Input: part model. Units: mm. Frame: model coordinates. Coordinates: 2 decimals unless noted, no trailing zeros. Write each loop counter-clockwise with the first axis right and the second up, starting at its lowest first coordinate (ties: lowest second). Pieces come first, ordered by that corner, then holes. Notation, with made-up numbers: M -11.75,19 L 14.25,19 A14 cw 14.25,37 Z; hole C -24,-26.5 d3. An arc over 180 degrees is marked long. Use one line per item in the form item = value.
from build123d import *

# Parameters (mm, degrees)
SKETCH6_W             = 25.4
SKETCH6_H             = 25.4
SKETCH6_W_2           = 20.32
SKETCH6_H_2           = 20.32
BOSS_EXTRUDE3_DEPTH   = 363.22
BOSS_EXTRUDE3_2_DEPTH = 363.22
SKETCH7_W             = 50.8
SKETCH7_H             = 25.359897542
SKETCH7_W_2           = 45.72
SKETCH7_H_2           = 20.279897542
BOSS_EXTRUDE4_DEPTH   = 114.3
CUT_EXTRUDE1_DEPTH    = 384.612481677
CUT_EXTRUDE2_DEPTH    = 384.612481677
CIRPATTERN1_COUNT     = 3
SKETCH12_R            = 3
CUT_EXTRUDE3_DEPTH    = 519.942549655
SKETCH13_R            = 87.5
BOSS_EXTRUDE6_DEPTH   = 2
SKETCH14_R            = 3
CUT_EXTRUDE4_DEPTH    = 518.180396616


with BuildPart() as part:
    # Sketch6 → Boss-Extrude3 (new body)
    with BuildSketch(Plane.XY.offset(-12.7)):
        with Locations((-44.45, 0)):
            Rectangle(SKETCH6_W, SKETCH6_H)
        with Locations((-44.45, 0)):
            Rectangle(SKETCH6_W_2, SKETCH6_H_2, mode=Mode.SUBTRACT)
    extrude(amount=-BOSS_EXTRUDE3_DEPTH)



with BuildPart() as body_2:
    # Sketch6 → Boss-Extrude3 2 (new body)
    with BuildSketch(Plane.XY.offset(-12.7)):
        with Locations((44.45, 0)):
            Rectangle(SKETCH6_W, SKETCH6_H)
        with Locations((44.45, 0)):
            Rectangle(SKETCH6_W_2, SKETCH6_H_2, mode=Mode.SUBTRACT)
    extrude(amount=-BOSS_EXTRUDE3_2_DEPTH)


with BuildPart() as part_1:
    add(part.part)

    add(body_2.part)  # Boss-Extrude4 merges body 2
    # Sketch7 → Boss-Extrude4 (add)
    with BuildSketch(Plane(origin=(-57.15, 0, 0), x_dir=(0, 0, -1), z_dir=(1, 0, 0))):
        with Locations((350.52, -25.379948771)):
            Rectangle(SKETCH7_W, SKETCH7_H)
        with Locations((350.52, -25.379948771)):
            Rectangle(SKETCH7_W_2, SKETCH7_H_2, mode=Mode.SUBTRACT)
    extrude(amount=BOSS_EXTRUDE4_DEPTH)

    # Sketch9 → Cut-Extrude1 (cut, through all)
    with BuildSketch(Plane(origin=(0, 12.7, 0), x_dir=(1, 0, 0), z_dir=(0, 1, 0))):
        Polygon((0, 0), (66.166370432, 38.20117178), (56.531711502, -13.195312554), align=None)
    extrude(amount=-CUT_EXTRUDE1_DEPTH, mode=Mode.SUBTRACT)

    # Sketch10 → Cut-Extrude2 (cut, through all)
    with BuildSketch(Plane(origin=(0, 12.7, 0), x_dir=(1, 0, 0), z_dir=(0, 1, 0))):
        Polygon((0, 0), (-91.357136084, 52.74506711), (-72.051101597, -19.306034487), align=None)
    extrude(amount=-CUT_EXTRUDE2_DEPTH, mode=Mode.SUBTRACT)


with BuildPart() as cirpattern1_1:
    # CirPattern1: pattern copy
    add(part_1.part.rotate(Axis((0, 0, 0), (0, 1, 0)), 1 * 360 / CIRPATTERN1_COUNT))


with BuildPart() as cirpattern1_2:
    # CirPattern1: pattern copy
    add(part_1.part.rotate(Axis((0, 0, 0), (0, 1, 0)), 2 * 360 / CIRPATTERN1_COUNT))


with BuildPart() as cut_extrude3_tool:
    # Sketch12 → Cut-Extrude3 (new, through all)
    with BuildSketch(Plane(origin=(0, 12.7, 0), x_dir=(1, 0, 0), z_dir=(0, 1, 0))):
        with Locations(Location((44.45, 40.327916303, 0), (0, 0, 90))):
            Circle(SKETCH12_R)
        with Locations(Location((57.15, 18.330871047, 0), (0, 0, 90))):
            Circle(SKETCH12_R)
    extrude(amount=-CUT_EXTRUDE3_DEPTH)


with BuildPart() as part_2:
    add(part_1.part)

    # Cut-Extrude3: cut by cut_extrude3_tool
    add(cut_extrude3_tool.part, mode=Mode.SUBTRACT)


    add(cirpattern1_1.part)  # Boss-Extrude6 merges CirPattern1_1


with BuildPart() as cirpattern1_2_1:
    add(cirpattern1_2.part)

    # Cut-Extrude3: cut by cut_extrude3_tool
    add(cut_extrude3_tool.part, mode=Mode.SUBTRACT)


with BuildPart() as part_3:
    add(part_2.part)

    add(cirpattern1_2_1.part)  # Boss-Extrude6 merges CirPattern1_2
    # Sketch13 → Boss-Extrude6 (add)
    with BuildSketch(Plane(origin=(0, 12.7, 0), x_dir=(1, 0, 0), z_dir=(0, 1, 0))):
        with Locations(Location((0, 0, 0), (0, 0, 68.724233024))):
            Circle(SKETCH13_R)
    extrude(amount=BOSS_EXTRUDE6_DEPTH)

    # Sketch14 → Cut-Extrude4 (cut, through all)
    with BuildSketch(Plane.XZ.offset(12.7)):
        with Locations(Location((57.15, -18.330871047, 0), (0, 0, 270))):
            Circle(SKETCH14_R)
        with Locations(Location((44.45, -40.327916303, 0), (0, 0, 270))):
            Circle(SKETCH14_R)
        with Locations(Location((-57.15, -18.330871047, 0), (0, 0, 270))):
            Circle(SKETCH14_R)
        with Locations(Location((-44.45, -40.327916303, 0), (0, 0, 270))):
            Circle(SKETCH14_R)
        with Locations(Location((12.7, 58.65878735, 0), (0, 0, 270))):
            Circle(SKETCH14_R)
        with Locations(Location((-12.7, 58.65878735, 0), (0, 0, 270))):
            Circle(SKETCH14_R)
        with Locations(Location((44.45, -65.727916303, 0), (0, 0, 270))):
            Circle(SKETCH14_R)
        with Locations(Location((79.147045256, -5.630871047, 0), (0, 0, 270))):
            Circle(SKETCH14_R)
        with Locations(Location((34.697045256, 71.35878735, 0), (0, 0, 270))):
            Circle(SKETCH14_R)
        with Locations(Location((-34.697045256, 71.35878735, 0), (0, 0, 270))):
            Circle(SKETCH14_R)
        with Locations(Location((-79.147045256, -5.630871047, 0), (0, 0, 270))):
            Circle(SKETCH14_R)
        with Locations(Location((-44.45, -65.727916303, 0), (0, 0, 270))):
            Circle(SKETCH14_R)
    extrude(amount=-CUT_EXTRUDE4_DEPTH, mode=Mode.SUBTRACT)


solid = part_3.part
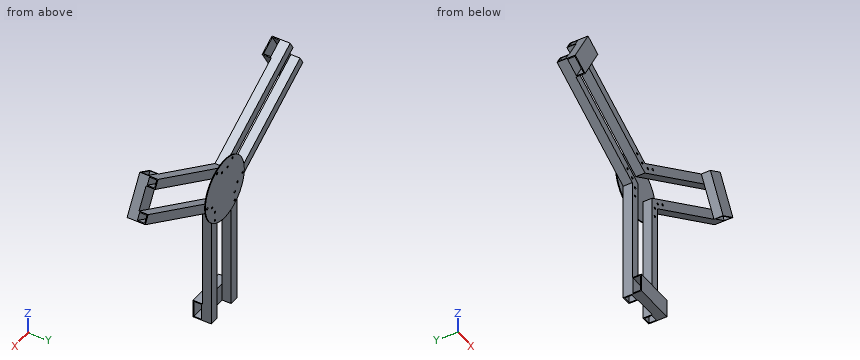
(1) Section query A-A on z = -120.5. Return the cut outline in (x, y), plus the area to 3 significant figures.
Computed:
outline = M -57.15,-12.7 L -31.75,-12.7 L -31.75,12.7 L -57.15,12.7 Z; M 31.75,-12.7 L 57.15,-12.7 L 57.15,12.7 L 31.75,12.7 Z; hole M -54.61,-10.16 L -34.29,-10.16 L -34.29,10.16 L -54.61,10.16 Z; hole M 34.29,-10.16 L 54.61,-10.16 L 54.61,10.16 L 34.29,10.16 Z
area = 465 mm^2
(2) First-contact query: pin 1 Ø5.5 at (x, z) = (-44.45, -40.33) entering from -Y; pin 2 Ø7 at (x, z) = (57.15, -18.33) entering from -Y; pin 3 Ø20.5 at (y, z) = (-0.5, -133) entering from -X; pin 4 Ø6 at (x, y) = (-9, -26) entering from +Z. Flat tips, straight axial feed; report the tip coordinate or a pass-through.
Computed:
pin_1 = through
pin_2 = -12.7
pin_3 = -57.15
pin_4 = -325.12
(3) Section query B-B on x = 123. Return the cut outline in (y, z).
Computed:
outline = M -12.7,5.02 L 12.7,5.02 L 12.7,34.35 L -12.7,34.35 Z; M -12.7,107.68 L 12.7,107.68 L 12.7,137.01 L -12.7,137.01 Z; hole M -10.16,7.96 L 10.16,7.96 L 10.16,31.42 L -10.16,31.42 Z; hole M -10.16,110.61 L 10.16,110.61 L 10.16,134.07 L -10.16,134.07 Z
(4) Line query: probe 1 along X at (y, z) = (-10, -204); probe 2 along Z at (x, y) = (129.5, 5). Output: solid intervals per line, ascending.
Computed:
probe_1 = -57.15 to -54.61, -34.29 to -31.75, 31.75 to 34.29, 54.61 to 57.15
probe_2 = 8.78 to 11.71, 35.17 to 38.11, 111.43 to 114.36, 137.83 to 140.76
